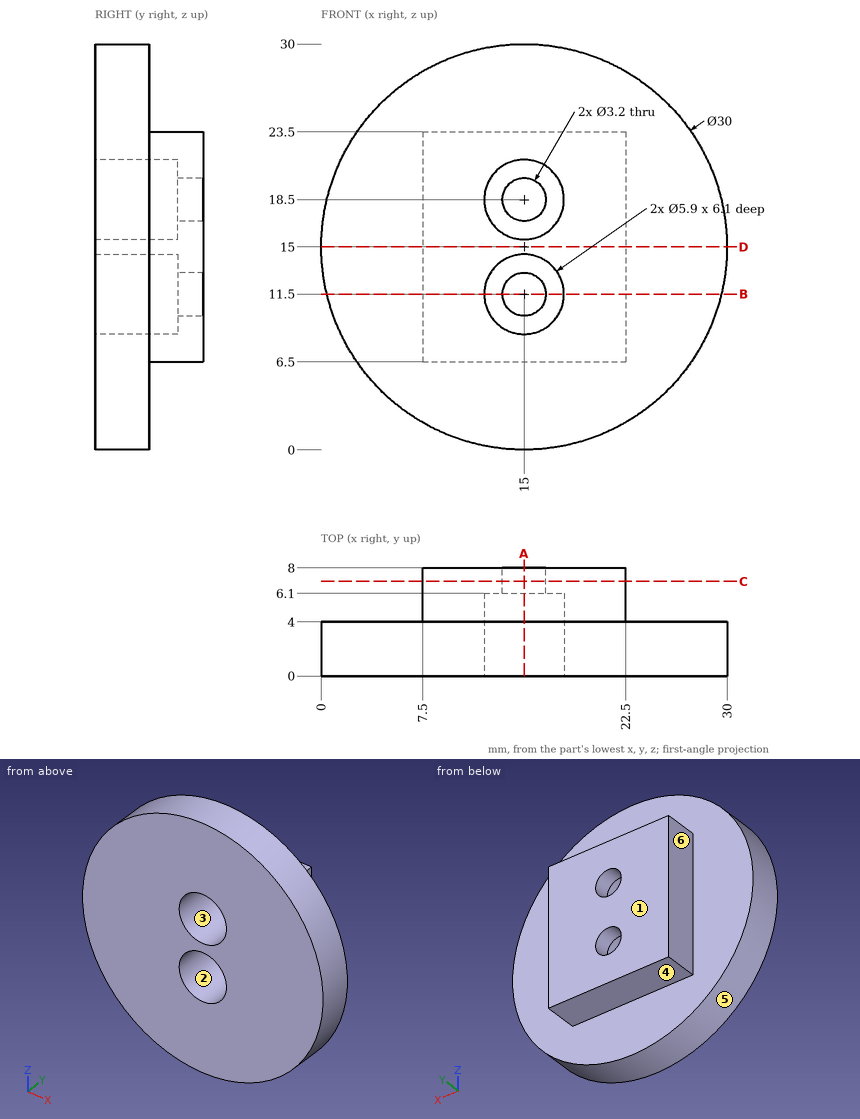
Input: dimensioned drawing with shaded views. Units: mm. Origin: part minimum x, y, z. A direction names the side the tool comes from. Give positions to 0.01 mm unless a question says otherwise; leave off trailing zeros. Loops run counter-clockwise (first coordinate to the right, second up) from the corner with the lowest first, then second, coordinate; pieces in that order, holes last. Notation, with made-up numbers: (0.25, 42.5) -> (38.25, 42.5) arc R25 ccw to (38.25, 73.5) -> close; hole circle Ø3 at (40, 4.5). An arc over 180 degrees is marked (long way). Use a Markdown table: item, result. Add a question column.
1) Reachability of the marked faces 1 and 2 from +Z, -Z, +X, -X, +Y, -Y: full face, straight path, thin tool, end or side. Return the list, or none.
2) Section query D-D, the plane z = 15. Return the cut outline in (x, y), then the cut area to 3 significant figures.
3) Section query A-A, the plane x = 15. Return the cut outline in (y, z), then the cut area to 3 significant figures.
4) First-contact query: pin 1 (1.2 mm diameter, centred on x = 16, y = 6.5, fed in from -Z); pin 2 (4.5 mm diameter, centred on y = 6, z = 17.5, fed in from -X); pin 3 (2 mm diameter, centred on x = 21.5, y = 3, fed in from -Z). Flat tips, straight axial feed; report the tip coordinate or a pass-through.
5) Pull-direction query (X, two-part tool) for the marked faces 3, 4, 5 and 6; classes: +X half, -X half, draft (parallel to the pull), parting line (faces both ways), or undercut.
6) Line query: line 1 along Z through (x, y) = (14.5, 3.75); line 2 along X through (y, z) = (7.25, 18.5); line 3 along Y through (x, z) = (3.75, 10.5). Output: solid intervals per line, ascending. Write a range as [from, to].
7) Section query B-B, the plane z = 11.5. Return the cut outline in (x, y).
8) Section query C-C, the plane y = 7. Return the cut outline in (x, z).
Numbers:
| question | item | result |
|---|---|---|
| 1 | face 1 | +Z, -Z, +X, -X, +Y |
| 1 | face 2 | -Y |
| 2 | outline | (0, 0) -> (30, 0) -> (30, 4) -> (22.5, 4) -> (22.5, 8) -> (7.5, 8) -> (7.5, 4) -> (0, 4) -> close |
| 2 | area | 180 mm2 |
| 3 | outline | (0, 0) -> (4, 0) -> (4, 6.5) -> (8, 6.5) -> (8, 9.9) -> (6.1, 9.9) -> (6.1, 8.55) -> (0, 8.55) -> close; (0, 14.45) -> (6.1, 14.45) -> (6.1, 13.1) -> (8, 13.1) -> (8, 16.9) -> (6.1, 16.9) -> (6.1, 15.55) -> (0, 15.55) -> close; (0, 21.45) -> (6.1, 21.45) -> (6.1, 20.1) -> (8, 20.1) -> (8, 23.5) -> (4, 23.5) -> (4, 30) -> (0, 30) -> close |
| 3 | area | 104 mm2 |
| 4 | pin 1 | stops at z = 6.5 |
| 4 | pin 2 | stops at x = 0.07 |
| 4 | pin 3 | stops at z = 1.04 |
| 5 | face 3 | undercut |
| 5 | face 4 | draft |
| 5 | face 5 | parting line |
| 5 | face 6 | -X half |
| 6 | line 1 | z = [0.01, 8.59], [14.41, 15.59], [21.41, 29.99] |
| 6 | line 2 | x = [7.5, 13.4], [16.6, 22.5] |
| 6 | line 3 | y = [0, 4] |
| 7 | outline | (0.41, 0) -> (12.05, 0) -> (12.05, 6.1) -> (13.4, 6.1) -> (13.4, 8) -> (7.5, 8) -> (7.5, 4) -> (0.41, 4) -> close; (16.6, 6.1) -> (17.95, 6.1) -> (17.95, 0) -> (29.59, 0) -> (29.59, 4) -> (22.5, 4) -> (22.5, 8) -> (16.6, 8) -> close |
| 8 | outline | (7.5, 6.5) -> (22.5, 6.5) -> (22.5, 23.5) -> (7.5, 23.5) -> close; hole circle Ø3.2 at (15, 11.5); hole circle Ø3.2 at (15, 18.5) |
